Could you check a few things on this model? Use its own coordinates, in mm. Face numbers are marked on the shaded views. A direction names the side the tool comes from. Give positions to 0.01 mm unless a question says otherwise; leave off trailing zeros. Write each loop counter-clockwise with the first axis right and the second up, starting at its lowest first coordinate (ties: lowest second). Pieces come first, ordered by that corner, then holes. Notation, with made-up numbers: M 77.25,33 L 118.25,33 A25 ccw 118.25,54 Z; hole C 44,-22.75 d7. An arc over 180 degrees is marked long. Write each question's results on one line, items separated by ' | '. Start each with the question number.
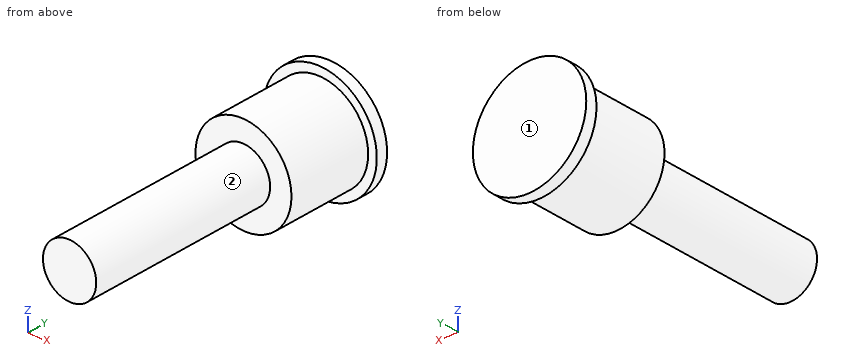
from build123d import *

# Parameters (mm, degrees)
F0_R     = 7.05
F1_DEPTH = 50.8
F2_R     = 12.7
F3_DEPTH = 25.4
F4_R     = 15
F5_DEPTH = 3


with BuildPart() as f1:
    # F0 (on Front) → F1 (new body)
    with BuildSketch(Plane.XZ):
        Circle(F0_R)
    extrude(amount=F1_DEPTH)

    # F2 (on Front) → F3 (join)
    with BuildSketch(Plane.XZ):
        Circle(F2_R)
    extrude(amount=-F3_DEPTH)

    # F4 (on face) → F5 (join)
    with BuildSketch(Plane(origin=(0, 25.4, 0), x_dir=(-1, 0, 0), z_dir=(0, 1, 0))):
        Circle(F4_R)
    extrude(amount=-F5_DEPTH)


solid = f1.part
Q1. If we section it at D-D (x = 11.5): Please give me the cut outline in (y, z), plus the area to 3 significant figures.
Q2. If we section it at B-B (x = 0): Please give me the cut outline in (y, z).
Q3. For the marked faces 1 and 2, which set-ups out of +Z, -Z, +X, -X, +Y, -Y let a thin tool reach every point of the face, with its end or its side?
Q4. If we section it at C-C (y = -5.5): Please give me the cut outline in (x, z).
Q5. I'm going to push flat-ended pins straight in: P1, Ø3, axis at y = -27, z = 2, coming from the -X side; P2, Ø12, axis at y = 14, z = -8, coming from the +X side; P3, Ø6, axis at x = -10.5, y = 15, coming from the -Z side. Where does each tip first touch, or does it pass through?
Q6. Please list where these lines run through material, in increasing order: line 1 (X direction, y = -23, z = -0.25); line 2 (Y direction, x = 8.75, z = -0.75); line 3 (Y direction, x = -4.5, z = 12). Write a range as [from, to].
Q7. If we section it at A-A (z = 0): Please give me the cut outline in (x, y).
Determined:
1) outline: M 0,-5.39 L 22.4,-5.39 L 22.4,-9.63 L 25.4,-9.63 L 25.4,9.63 L 22.4,9.63 L 22.4,5.39 L 0,5.39 Z | area: 299 mm²
2) outline: M -50.8,-7.05 L 0,-7.05 L 0,-12.7 L 22.4,-12.7 L 22.4,-15 L 25.4,-15 L 25.4,15 L 22.4,15 L 22.4,12.7 L 0,12.7 L 0,7.05 L -50.8,7.05 Z
3) face 1: +Z, -Z, +X, -X, +Y | face 2: -Y
4) outline: C 0,0 d14.1
5) P1: stops at x = -7.03 | P2: stops at x = 12.54 | P3: stops at z = -10.25
6) line 1: x = [-7.05, 7.05] | line 2: y = [0, 25.4] | line 3: y = [22.4, 25.4]
7) outline: M -15,22.4 L -12.7,22.4 L -12.7,0 L -7.05,0 L -7.05,-50.8 L 7.05,-50.8 L 7.05,0 L 12.7,0 L 12.7,22.4 L 15,22.4 L 15,25.4 L -15,25.4 Z
